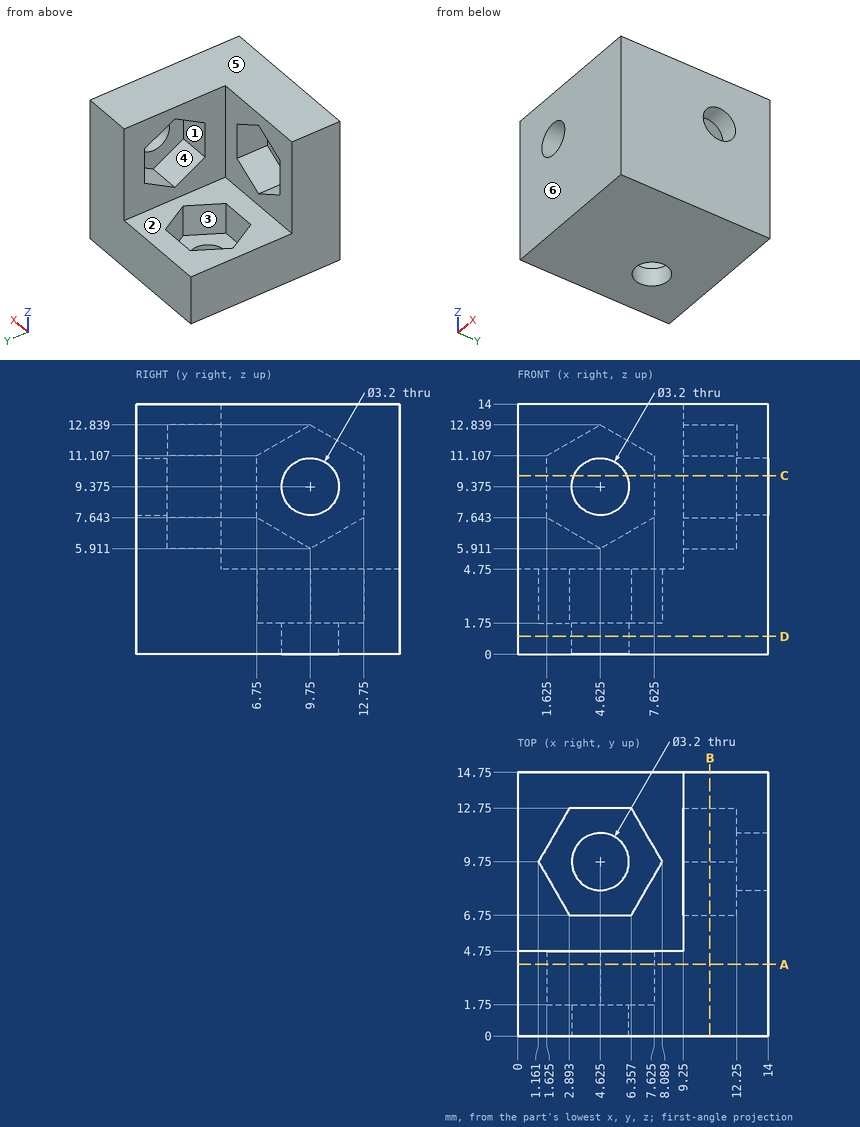
The figure shows three views and two pictorial views of one solid part (mm, origin at its lowest corner). Answer the questions. A direction names the side the tool comes from. Round coordinates to 2 decimals unless told otherwise and drop trailing zeros. Write each loop counter-clockwise with the first axis right and the second up, starting at its lowest first coordinate (ties: lowest second). Pieces come first, ordered by that corner, then holes. Notation, with made-up numbers: M -3,4.5 L 44,4.5 A8 cw 44,14.5 Z; hole C -6.5,-16.75 d7. An arc over 180 degrees is marked long. Use a Markdown table: item, result.
1) The part is cut by section A-A on y = 4. Give the vertices of the cut face in (x, z) (3 decimals), plus the area to 3 significant figures.
Taken from the geometry:
| item | result |
|---|---|
| outline | M 0,0 L 14,0 L 14,14 L 0,14 Z; hole M 1.625,7.643 L 4.625,5.911 L 7.625,7.643 L 7.625,11.107 L 4.625,12.839 L 1.625,11.107 Z |
| area | 165 mm2 |
2) Which of the six approach directions +Z, -Z, +X, -X, +Y, -Y give full straight-line access (tool end or side, diameter ignored) to the marked faces 1, 2 and 3?
Taken from the geometry:
| item | result |
|---|---|
| face 1 | -X |
| face 2 | +Z, -X, +Y |
| face 3 | +Z |
3) The part is cut by section D-D on z = 1. Give the vertices of the cut face in (x, y) (3 decimals), plus the area to 3 significant figures.
Taken from the geometry:
| item | result |
|---|---|
| outline | M 0,0 L 14,0 L 14,14.75 L 0,14.75 Z; hole C 4.625,9.75 d3.2 |
| area | 198 mm2 |
4) The part is cut by section B-B on x = 10.75. Give the vertices of the cut face in (y, z), plus the area to 3 significant figures.
Taken from the geometry:
| item | result |
|---|---|
| outline | M 0,0 L 14.75,0 L 14.75,14 L 0,14 Z; hole M 6.75,7.64 L 9.75,5.91 L 12.75,7.64 L 12.75,11.11 L 9.75,12.84 L 6.75,11.11 Z |
| area | 175 mm2 |
5) Flat-ended cylindrical pins translate along their axes: pin 1 (2.5 mm diameter, centred on x = 5, z = 4, fed in from -Y); pin 2 (2.5 mm diameter, centred on y = 9.75, z = 9.375, fed in from +X); pin 3 (4 mm diameter, centred on y = 7.5, z = 9, fed in from -X); pin 4 (4.5 mm diameter, centred on x = 3.5, y = 9.5, fed in from +Z). Find the tip coordinate at first contact, or state that the pin passes through.
Taken from the geometry:
| item | result |
|---|---|
| pin 1 | stops at y = 0 |
| pin 2 | passes through |
| pin 3 | stops at x = 9.25 |
| pin 4 | stops at z = 4.75 |
6) Consider line 1 (Z direction, x = 13.1, y = 9.75) (3 decimals); line 2 (Y direction, x = 9.75, z = 9.25); line 3 (X direction, y = 12.5, z = 10). Determine where each line is inside the solid, lowest interval first. Write a range as [from, to].
Taken from the geometry:
| item | result |
|---|---|
| line 1 | z = [0, 7.775], [10.975, 14] |
| line 2 | y = [0, 6.75], [12.75, 14.75] |
| line 3 | x = [12.25, 14] |
7) The part is cut by section C-C on z = 10. Give the vertices of the cut face in (x, y) (3 decimals).
Taken from the geometry:
| item | result |
|---|---|
| outline | M 0,0 L 3.152,0 L 3.152,1.75 L 1.625,1.75 L 1.625,4.75 L 0,4.75 Z; M 6.098,0 L 14,0 L 14,8.277 L 12.25,8.277 L 12.25,6.75 L 9.25,6.75 L 9.25,4.75 L 7.625,4.75 L 7.625,1.75 L 6.098,1.75 Z; M 9.25,12.75 L 12.25,12.75 L 12.25,11.223 L 14,11.223 L 14,14.75 L 9.25,14.75 Z |
8) Determine the mould class of the marked faces 4, 5 and 6 for opening direction Z: pulls with the +Z half, pulls with the -Z half, needs draft (parallel to the pull), parting line crosses it, or undercut.
Taken from the geometry:
| item | result |
|---|---|
| face 4 | undercut |
| face 5 | pulls with the +Z half |
| face 6 | needs draft |
